For this review, take the finished solid that the model builds, in its own axes (mm). Round coordinates to 2 decimals unless told otherwise and drop trailing zeros. Write each loop counter-clockwise with the first axis right and the second up, starting at its lowest first coordinate (ties: lowest second). Pieces come first, ordered by that corner, then holes. Notation, with made-up numbers: (-40, -39) -> (-15, -39) arc R29 cw to (-15, -15) -> close; hole circle Ø7 at (46.5, -22). An arc over 180 degrees is marked (long way). Write each question's results on one line, items separated by ' | '. Start each with the question number.
Item 1: Add section C-C (z = 12). State the section outline as (x, y) points, plus the area to 3 significant figures.
Item 2: To check wall thickness, follow line 1 along X through (y, z) = (-0.15, 8.5); line 2 along Z through (x, y) = (0.25, -2.1); line 3 along X through (y, z) = (1.4, 4.75). State the ranges of each line that lie inside material, in increasing order.
Item 3: Add section A-A (y = 0). State the section outline as (x, z) points, plus the area to 3 significant figures.
Item 4: Add section B-B (x = 0). State the section outline as (y, z) points, plus the area to 3 significant figures.
Item 5: Clearance check with flat-ended pins moving along their axes: pin 1 (1.2 mm diameter, centred on y = 0.5, z = 14, fed in from +X); pin 2 (1 mm diameter, centred on x = 2, z = 11.5, fed in from -Y); pin 3 (0.5 mm diameter, centred on x = 0, y = 0.5, fed in from +Z). State where each tip first meets the part, or that it passes through.
from build123d import *

# Parameters (mm, degrees)
SKETCH_1_R          = 3
EXTRUDE_1_DEPTH     = 15
CHAMFER_1_SIZE      = 0.5545
SKETCH_2_W          = 0.6
SKETCH_2_H          = 7
CUT_EXTRUDE_1_DEPTH = 1.5


with BuildPart() as part:
    # Эскиз1 → Бобышка-Вытянуть1 (new body)
    with BuildSketch(Plane.XY):
        Circle(SKETCH_1_R)
    extrude(amount=EXTRUDE_1_DEPTH)

    # Фаска1
    chamfer_1_edges = [part.edges().sort_by_distance(p)[0] for p in [
        (-3, 0, 0),
        (-3, 0, 15),
    ]]
    chamfer(chamfer_1_edges, length=CHAMFER_1_SIZE)

    # Эскиз2 → Вырез-Вытянуть1 (cut)
    with BuildSketch(Plane.XY.offset(15)):
        Rectangle(SKETCH_2_W, SKETCH_2_H)
    extrude(amount=-CUT_EXTRUDE_1_DEPTH, mode=Mode.SUBTRACT)


solid = part.part
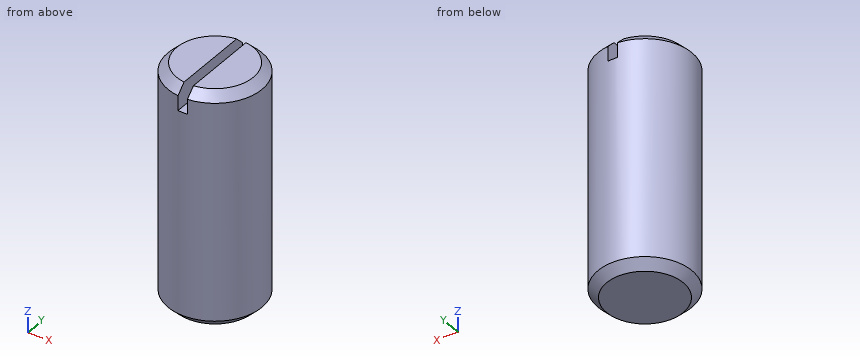
Responses:
1) outline: circle Ø6 at (0, 0) | area: 28.3 mm^2
2) line 1: x = -3 to 3 | line 2: z = 0 to 13.5 | line 3: x = -2.65 to 2.65
3) outline: (-3, 0.55) -> (-2.45, 0) -> (2.45, 0) -> (3, 0.55) -> (3, 14.45) -> (2.45, 15) -> (0.3, 15) -> (0.3, 13.5) -> (-0.3, 13.5) -> (-0.3, 15) -> (-2.45, 15) -> (-3, 14.45) -> close | area: 88.5 mm^2
4) outline: (-3, 0.55) -> (-2.45, 0) -> (2.45, 0) -> (3, 0.55) -> (3, 13.5) -> (-3, 13.5) -> close | area: 80.7 mm^2
5) pin 1: stops at x = 3 | pin 2: stops at y = -2.6 | pin 3: stops at z = 13.5
